Autodesk Inventor part; units mm, degrees
ref_plane "YZ Plane" through (0, 0, 0) normal (1, 0, 0) x (0, 1, 0)
ref_plane "XZ Plane" through (0, 0, 0) normal (0, 1, 0) x (-1, 0, 0)
ref_plane "XY Plane" through (0, 0, 0) normal (0, 0, 1) x (1, 0, 0)
sketch "Sketch1" plane through (0, 0, 0) normal (0, 0, 1) x (1, 0, 0)
  line L0 (10.25, -111.5) -> (-10.25, -111.5)
  line L1 (-10.25, -111.5) -> (-10.25, 111.5)
  line L2 (-10.25, 111.5) -> (10.25, 111.5)
  line L3 (10.25, 111.5) -> (10.25, -111.5)
  line L4 (10.25, -111.5) -> (-10.25, 111.5) construction
  line L5 (-10.25, -111.5) -> (10.25, 111.5) construction
  line L6 (-2.25, 103.5) -> (-2.25, -103.5) construction
  point P0 (0, 0)
  point P1 (-2.25, 34.5)
  point P2 (-2.25, -34.5)
  point P3 (-2.25, 0)
  dimension "d0" = 20.5
  dimension "d4" = 69
  dimension "d9" = 8
  dimension "d10" = 8
extrude "Extrusion1" add sketch "Sketch1" against normal blind 14
fillet "Fillet1" radius 4 2 edges at (-10.25, 111.5, -7) (-10.25, -111.5, -7)
chamfer "Chamfer1" distance 2 angle 45 5 edges at (2, 111.5, -14) (-9.0784, 110.3284, -14) (-10.25, 0, -14) (-9.0784, -110.3284, -14) (2, -111.5, -14)
hole "Hole1" at (-2.25, 103.5, 0) at (-2.25, 34.5, 0) at (-2.25, -34.5, 0) at (-2.25, -103.5, 0) direction (0, 0, -1) diameter 6.5 end through all
sketch "Sketch2" plane through (-10.25, -107.5, 0) normal (-1, 0, 0) x (0, 0, 1)
  line L0 (-6, 197.5) -> (-6, 17.5) construction
  line L1 (0, 215) -> (0, 0)
  point P0 (0, 107.5)
  point P1 (0, 107.5)
  point P2 (-6, 107.5)
  point P3 (-6, 107.5)
  dimension "d24" = 180
  dimension "d25" = 6
hole "Hole2" at (-10.25, 90, -6) at (-10.25, 0, -6) at (-10.25, -90, -6) direction (1, 0, 0) diameter 5.4 end through all counterbore diameter 9.5 counterbore depth 6.5
chamfer "Chamfer2" distance 1 angle 45 4 edges at (-2.25, -100.25, 0) (-2.25, -31.25, 0) (-2.25, 37.75, 0) (-2.25, 106.75, 0)
equation "\"d10\" = d9"
properties part number "Door Bar Front Panel Mount" material "ABS Plastic"
Check sheet for the modelled part. Datum: model origin and axes. Units: mm. A direction names the side the tool comes from. Give positions to 0.01 mm unless a question says otherwise; leave off trailing zeros. Write each loop counter-clockwise with the first axis right and the second up, starting at its lowest first coordinate (ties: lowest second). Pieces come first, ordered by that corner, then holes. Notation, with made-up numbers: (-16, -38.5) -> (-2, -38.5) arc R16 ccw to (-2, -30.5) -> close; hole circle Ø8 at (10, -27.5). An arc over 180 degrees is marked (long way). Use CSV: the item, a comma, the result in double quotes. Start each with the question number.
Q1. Cross-section at B-B on y = -103.5. Enter the section's corners in (x, z), and give its area (3 significant figures).
Q2. Release check for a two-part mould opening along Z. For faces 3 (the flat face through (1, 2, -14)), 4 (the flat face through (-3.75, -87.96, -3.96)), 5 (the cylindrical face through (-3.23, 31.4, -7.59)) record: +Z half, -Z half, draft (parallel to the pull), parting line (faces both ways), or undercut.
Q3. Scan lines: line 1 along Y through (x, z) = (-6.5, -6); line 2 along Z through (x, y) = (-7.75, 90); line 3 along Y through (x, z) = (-4.75, -12.25). Record each from-to range of solid material in increasing order.
Q4. Cross-section at C-C on x = 5. Enter the section's corners in (y, z).
Q5. Tool access check on faces 1 (the cylindrical face through (3.348, -0.811, -3.425)), 2 (the cylindrical face through (-6.954, 4.637, -7.03)). Record the directions out of +Z, -Z, +X, -X, +Y, -Y that give a thin tool (end or side, any length) a straight path to the whole face; none if there is none.
Q6. Depth check by flat-ended pin: P1, Ø4.5, axis at y = -90, z = -6, coming from the -X side; P2, Ø7.5, axis at y = -90, z = -6, coming from the -X side; P3, Ø10.5, axis at x = -2.25, y = -34.5, coming from the +Z side. Enter the tip coordinate at first touch or a pass-through.
Q7. Cross-section at A-A on z = -6. Count the separate pieces of the cut face and the enclosed holes in it, and give its area (3 significant figures).
Q8. Cross-section at D-D on y = 90. Enter the section's corners in (x, z), and give its area (3 significant figures).
Working result:
1,outline,"(-10.25, -12) -> (-8.25, -14) -> (-5.5, -14) -> (-5.5, -1) -> (-6.5, 0) -> (-10.25, 0) -> close; (1, -14) -> (10.25, -14) -> (10.25, 0) -> (2, 0) -> (1, -1) -> close"
1,area,"193 mm^2"
2,face 3,"-Z half"
2,face 4,"undercut"
2,face 5,"draft"
3,line 1,"y = -111.49 to -94.75, -85.25 to -4.75, 4.75 to 85.25, 94.75 to 111.49"
3,line 2,"z = -14 to -10.75, -1.25 to 0"
3,line 3,"y = -111.25 to -105.58, -101.42 to -36.58, -32.42 to 32.42, 36.58 to 101.42, 105.58 to 111.25"
4,outline,"(-111.5, -12) -> (-109.5, -14) -> (109.5, -14) -> (111.5, -12) -> (111.5, 0) -> (-111.5, 0) -> close; hole circle Ø5.4 at (-90, -6); hole circle Ø5.4 at (0, -6); hole circle Ø5.4 at (90, -6)"
5,face 1,"+X, -X"
5,face 2,"-X"
6,P1,"passes through"
6,P2,"stops at x = -3.75"
6,P3,"stops at z = 0"
7,separate pieces,"4"
7,enclosed holes,"4"
7,area,"4,020 mm^2"
8,outline,"(-10.25, -12) -> (-8.25, -14) -> (10.25, -14) -> (10.25, -8.7) -> (-3.75, -8.7) -> (-3.75, -10.75) -> (-10.25, -10.75) -> close; (-10.25, -1.25) -> (-3.75, -1.25) -> (-3.75, -3.3) -> (10.25, -3.3) -> (10.25, 0) -> (-10.25, 0) -> close"
8,area,"148 mm^2"
